```python
from build123d import *

# Parameters (mm, degrees)
BOSS_EXTRUDE1_DEPTH = 35
SKETCH9_R           = 5
BOSS_EXTRUDE3_DEPTH = 15
SKETCH10_W          = 39.744762059
SKETCH10_H          = 6.949903748
CUT_EXTRUDE1_DEPTH  = 13
SKETCH11_R          = 0.5
CUT_EXTRUDE2_DEPTH  = 47.286707872
SKETCH12_R          = 3
CUT_EXTRUDE3_DEPTH  = 53.72991015


with BuildPart() as part:
    # Sketch4 → Boss-Extrude1 (new, symmetric)
    with BuildSketch(Plane.XY):
        with BuildLine():
            Line((7.5, -2.9), (-7.5, -2.9))
            ThreePointArc((-7.5, -2.9), (-10.4, 0), (-7.5, 2.9))
            Line((-7.5, 2.9), (7.5, 2.9))
            ThreePointArc((7.5, 2.9), (10.4, 0), (7.5, -2.9))
        make_face()
        with BuildLine():
            Line((7.5, -1.9), (-7.5, -1.9))
            ThreePointArc((-7.5, -1.9), (-9.4, 0), (-7.5, 1.9))
            Line((-7.5, 1.9), (7.5, 1.9))
            ThreePointArc((7.5, 1.9), (9.4, 0), (7.5, -1.9))
        make_face(mode=Mode.SUBTRACT)
    extrude(amount=BOSS_EXTRUDE1_DEPTH, both=True)

    # Sketch9 → Boss-Extrude3 (add, symmetric)
    with BuildSketch(Plane(origin=(0, 0, 0), x_dir=(0, 0, -1), z_dir=(1, 0, 0))):
        with Locations((-39.073082371, 0.015275052)):
            Circle(SKETCH9_R)
    extrude(amount=BOSS_EXTRUDE3_DEPTH, both=True)

    # Sketch10 → Cut-Extrude1 (cut, symmetric)
    with BuildSketch(Plane(origin=(0, 0, 0), x_dir=(1, 0, 0), z_dir=(0, 1, 0))):
        with Locations((-2.189570447, -46.548034245)):
            Rectangle(SKETCH10_W, SKETCH10_H)
    extrude(amount=CUT_EXTRUDE1_DEPTH, both=True, mode=Mode.SUBTRACT)

    # Sketch11 → Cut-Extrude2 (cut, through all)
    with BuildSketch(Plane(origin=(0, 2.9, 0), x_dir=(1, 0, 0), z_dir=(0, 1, 0))):
        with Locations(Location((0, -26.870162273, 0), (0, 0, 180))):
            Circle(SKETCH11_R)
    extrude(amount=-CUT_EXTRUDE2_DEPTH, mode=Mode.SUBTRACT)

    # Sketch12 → Cut-Extrude3 (cut, through all)
    with BuildSketch(Plane(origin=(15, 0, 0), x_dir=(0, 0, -1), z_dir=(1, 0, 0))):
        with Locations((-39.073082371, 0.015275052)):
            Circle(SKETCH12_R)
    extrude(amount=-CUT_EXTRUDE3_DEPTH, mode=Mode.SUBTRACT)


solid = part.part
```
Work out the finished part from the listing and answer in its coordinate system (mm). A direction names the side the tool comes from. Give positions to 0.01 mm unless a question says otherwise; leave off trailing zeros. Loops run counter-clockwise (first coordinate to the right, second up) from the corner with the lowest first, then second, coordinate; pieces in that order, holes last. Notation, with made-up numbers: (55, 37) - (90, 37) arc R27 cw to (90, 73) - close; hole circle Ø9 at (-8, -22.75). An arc over 180 degrees is marked (long way). Use CSV: the item, a comma, the result in double quotes. Start each with the question number.
(1) Each of these flat-tipped pins is pushed along its axis until it touches: pin 1 (1 mm diameter, centred on y = 1, z = -25, fed in from +X); pin 2 (6 mm diameter, centred on y = 2, z = 31.5, fed in from +X); pin 3 (1.5 mm diameter, centred on x = 7.5, z = 11.5, fed in from -Y); pin 4 (12 mm diameter, centred on x = -1.5, z = -5.5, fed in from +Y). Where does it stop, or does it pass through?
(2) Determine the mould class of faces 4 (the face through (0, -2.9, 0)), 5 (the face through (15, 2.3, 36.6)), 6 (the face through (-9.4, 0, 0.2)) for opening direction X: released by +X, released by -X, zero draft, split by the parting line, or undercut.
(3) Find the intervals of material crossed by L1, parallel to Y at x = 9, z = 39; L2, parallel to Z at x = 0, y = -2.2; L3, parallel to Z at x = 11, y = 0, in increasing order.
(4) A tool of negligible diameter and unlimited length cuts with its end or side. For faces 1 (the face through (10.4, 0.1, 0.5)), 2 (the face through (0, -1.9, 0)), 3 (the face through (0, 2.9, 0)), from which of +Z, -Z, +X, -X, +Y, -Y can it reach the whole face along a straight path? Write none if from no direction.
(5) Find section A-A, the plane z = -24. Determine the outline of the cut face in (x, y), plus the area to 3 significant figures.
(6) Find section C-C, the plane y = 4. Determine the outline of the cut face in (x, z), plus the area to 3 significant figures.
Results found:
1,pin 1,"x = 10.36"
1,pin 2,"x = 15"
1,pin 3,"y = -2.9"
1,pin 4,"y = 2.9"
2,face 4,"zero draft"
2,face 5,"released by +X"
2,face 6,"undercut"
3,L1,"-4.98 to -2.98, 3.01 to 5.01"
3,L2,"-35 to 26.37, 27.37 to 37.05, 41.1 to 43.07"
3,L3,"34.07 to 36.07, 42.07 to 43.07"
4,face 1,"-Z, +X"
4,face 2,"-Z"
4,face 3,"-Z, +X, -X, +Y"
5,outline,"(-7.5, -2.9) - (7.5, -2.9) arc R2.9 ccw to (7.5, 2.9) - (-7.5, 2.9) arc R2.9 ccw to start; hole (-7.5, -1.9) - (7.5, -1.9) arc R1.9 ccw to (7.5, 1.9) - (-7.5, 1.9) arc R1.9 ccw to start"
5,area,"45.1 mm^2"
6,outline,"(-15, 36.05) - (15, 36.05) - (15, 42.09) - (-15, 42.09) - close"
6,area,"181 mm^2"
